Job drawing, mm, ordinate dimensions from the low corner. One solid piece. A direction names the side the tool comes from. Round coordinates to 2 decimals unless told otherwise and drop trailing zeros. Write each loop counter-clockwise with the first axis right and the second up, starting at its lowest first coordinate (ties: lowest second). Pieces come first, ordered by that corner, then holes.
1) Pull direction X, two halves, no side cores. Call the marked faces 3 and 4: +X half, -X half, draft (parallel to the pull), parting line (faces both ways), or undercut.
2) Saw through at C-C (z = 98.5). Write the cut outline in (x, y), plus the area to 3 significant figures.
3) Wall check: probe 1 along X at (y, z) = (5.5, 136); probe 2 along Z at (x, y) = (57.5, 9.5); probe 3 along X at (y, z) = (4.25, 75). Give the ranges that are in metal, low to high.
4) Saw through at B-B (x = 69). Write the cut outline in (y, z) (3 decimals), plus the area to 3 significant figures.
5) Saw through at A-A (z = 142.5). Write the cut outline in (x, y).
6) Flat gauge pins, fed straight in: pin 1 (3 mm diameter, centred on y = 6, z = 24, fed in from -X); pin 2 (3 mm diameter, centred on x = 64, y = 10.5, fed in from -Z); pin 3 (5.5 mm diameter, centred on y = 6.35, z = 153.416, fed in from -X); pin 4 (7.5 mm diameter, centred on y = 6.35, z = 6.35, fed in from +X). Where does each tip first touch, or does it go through?
7) Saw through at D-D (x = 53.5). Write the cut outline in (y, z), plus the area to 3 significant figures.
8) Which spindle directions (+Z, -Z, +X, -X, +Y, -Y) get a long thin tool onto all of the face, cutting with end or side? Do the marked faces 1 and 2. Say none if no direction does.
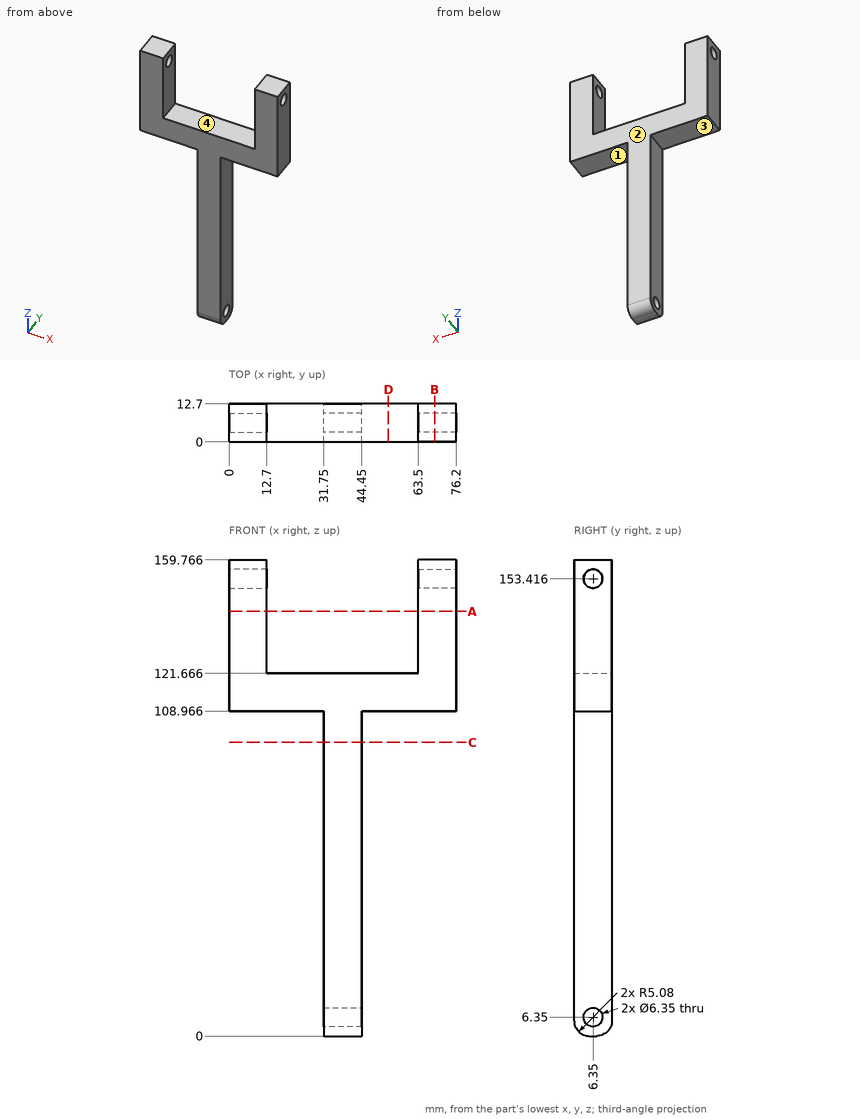
Evaluation:
1. face 3: draft
1. face 4: undercut
2. outline: (31.75, 0) - (44.45, 0) - (44.45, 12.7) - (31.75, 12.7) - close
2. area: 161 mm2
3. probe 1: x = 0 to 12.7, 63.5 to 76.2
3. probe 2: z = 108.97 to 121.67
3. probe 3: x = 31.75 to 44.45
4. outline: (0, 108.966) - (12.7, 108.966) - (12.7, 159.766) - (0, 159.766) - close; hole circle Ø6.35 at (6.35, 153.416)
4. area: 613 mm2
5. outline: (0, 0) - (12.7, 0) - (12.7, 12.7) - (0, 12.7) - close; (63.5, 0) - (76.2, 0) - (76.2, 12.7) - (63.5, 12.7) - close
6. pin 1: stops at x = 31.75
6. pin 2: stops at z = 108.97
6. pin 3: passes through
6. pin 4: stops at x = 44.45
7. outline: (0, 108.97) - (12.7, 108.97) - (12.7, 121.67) - (0, 121.67) - close
7. area: 161 mm2
8. face 1: -Z, +X, +Y, -Y
8. face 2: +Z, -Z, +X, -X, +Y
